from build123d import *

# Parameters (mm, degrees)
SCHIZZO1_W                   = 50
SCHIZZO1_H                   = 30
ESTRUSIONE_ESTRUSIONE1_DEPTH = 6
SCHIZZO2_R                   = 4
TAGLIO_ESTRUSIONE1_DEPTH     = 42.646332289
SCHIZZO3_R                   = 1.7
TAGLIO_ESTRUSIONE2_DEPTH     = 10


with BuildPart() as part:
    # Schizzo1 → Estrusione-Estrusione1 (new body)
    with BuildSketch(Plane(origin=(0, 0, 0), x_dir=(1, 0, 0), z_dir=(0, 1, 0))):
        with Locations((3.256273518, 0.703517588)):
            Rectangle(SCHIZZO1_W, SCHIZZO1_H)
    extrude(amount=ESTRUSIONE_ESTRUSIONE1_DEPTH)

    # Schizzo2 → Taglio-Estrusione1 (cut, through all)
    with BuildSketch(Plane.XY.offset(14.296482412)):
        with Locations((3.256273518, 6)):
            Circle(SCHIZZO2_R)
    extrude(amount=-TAGLIO_ESTRUSIONE1_DEPTH, mode=Mode.SUBTRACT)

    # Schizzo3 → Taglio-Estrusione2 (cut)
    with BuildSketch(Plane.XZ):
        with Locations(Location((-17.743726482, 10.296482412, 0), (0, 0, 270))):
            Circle(SCHIZZO3_R)
        with Locations(Location((24.256273518, 10.296482412, 0), (0, 0, 90))):
            Circle(SCHIZZO3_R)
        with Locations(Location((24.256273518, -11.703517588, 0), (0, 0, 270))):
            Circle(SCHIZZO3_R)
        with Locations(Location((-17.743726482, -11.703517588, 0), (0, 0, 90))):
            Circle(SCHIZZO3_R)
    extrude(amount=-TAGLIO_ESTRUSIONE2_DEPTH, mode=Mode.SUBTRACT)


solid = part.part
Can you work these out from the model? Positions are in its coordinate system, mm. Round coordinates to 2 decimals unless told otherwise and drop trailing zeros. Loops run counter-clockwise (first coordinate to the right, second up) from the corner with the lowest first, then second, coordinate; pieces in that order, holes last. Notation, with made-up numbers: (-15, 80.25) - (18, 80.25) arc R34 ccw to (18, 115.25) - close; hole circle Ø8 at (64.5, 46). An arc over 180 degrees is marked (long way). Answer in a Markdown table with one row per item. Add a question column.
Q1. For pin 1 Ø2 at (x, z) = (24.26, 10.3) entering from -Y, with a flat end and sliding along its axis, tell me the tip position at first contact or that it passes through.
Q2. I want a section at C-C on z = -10.5. List the corners of the cut face in (x, y) for me.
Q3. I want a section at B-B on z = 0.5. List the corners of the cut face in (x, y) for me.
Q4. I need wall thicknesses on L1, parallel to X at y = 3.75, z = -10.75; L2, parallel to X at y = 1.75, z = -11; L3, parallel to X at y = 5.75, z = 6.5. Which ranges of each line are inside material? Lowest first, please.
Q5. We'd pull the mould along X, two halves only. Please class faces 1 (the cylindrical face through (3.2, 2, -0.5)), 2 (the flat face through (28.256, 3, 0)), 3 (the flat face through (2.9, 1.6, 14.296)), 4 (the cylindrical face through (-19.403, 2.958, 10.665)): pulls with the +X half, pulls with the -X half, needs draft (parallel to the pull), parting line crosses it, or undercut.
Q6. I want a section at A-A on y = 4.5. List the corners of the cut face in (x, z) for me.
A:
| question | item | result |
|---|---|---|
| 1 | pin 1 | through |
| 2 | outline | (-21.74, 0) - (-18.94, 0) - (-18.94, 6) - (-21.74, 6) - close; (-16.54, 0) - (23.06, 0) - (23.06, 6) - (7.26, 6) arc R4 cw to (-0.74, 6) - (-16.54, 6) - close; (25.46, 0) - (28.26, 0) - (28.26, 6) - (25.46, 6) - close |
| 3 | outline | (-21.74, 0) - (28.26, 0) - (28.26, 6) - (7.26, 6) arc R4 cw to (-0.74, 6) - (-21.74, 6) - close |
| 4 | L1 | -21.74 to -19.15, -16.34 to -0.05, 6.56 to 22.85, 25.66 to 28.26 |
| 4 | L2 | -21.74 to -19.29, -16.2 to 22.71, 25.8 to 28.26 |
| 4 | L3 | -21.74 to -0.74, 7.25 to 28.26 |
| 5 | face 1 | undercut |
| 5 | face 2 | pulls with the +X half |
| 5 | face 3 | needs draft |
| 5 | face 4 | undercut |
| 6 | outline | (-21.74, -15.7) - (-0.45, -15.7) - (-0.45, 14.3) - (-21.74, 14.3) - close; (6.96, -15.7) - (28.26, -15.7) - (28.26, 14.3) - (6.96, 14.3) - close; hole circle Ø3.4 at (-17.74, -11.7); hole circle Ø3.4 at (-17.74, 10.3); hole circle Ø3.4 at (24.26, -11.7); hole circle Ø3.4 at (24.26, 10.3) |
